CAD build for the part. Positions are in the model's coordinates, mm. A direction names the side the tool comes from. Coordinates: 2 decimals unless noted, no trailing zeros. Write each loop counter-clockwise with the first axis right and the second up, starting at its lowest first coordinate (ties: lowest second). Pieces come first, ordered by that corner, then holes. Notation, with made-up numbers: M 32.5,57.5 L 43.5,57.5 A19 cw 43.5,90.5 Z; hole C 52,47.25 d2. An arc over 180 degrees is marked long. Put each result on its own line as item: value. Start each with the question number.
Autodesk Inventor part; units mm, degrees
ref_plane "YZ Plane" through (0, 0, 0) normal (1, 0, 0) x (0, 1, 0)
ref_plane "XZ Plane" through (0, 0, 0) normal (0, 1, 0) x (-1, 0, 0)
ref_plane "XY Plane" through (0, 0, 0) normal (0, 0, 1) x (1, 0, 0)
sketch "Эскиз1" plane through (0, 0, 0) normal (1, 0, 0) x (0, 1, 0)
  line L0 (0, 0) -> (0, -73.7994) construction
  line L1 (23.5, 0) -> (23.5, -65.8206)
  line L2 (23.5, -65.8206) -> (67.6779, -115.777)
  line L3 (125, -110.9688) -> (125, -104.777)
  line L4 (125, -104.777) -> (67.2948, -104.777)
  line L5 (67.2948, -104.777) -> (40.0448, -73.9627)
  line L6 (27.5, -40.8401) -> (27.5, -5)
  line L7 (27.5, -5) -> (32.5, -5)
  line L8 (32.5, -5) -> (32.5, 0)
  line L9 (32.5, 0) -> (23.5, 0)
  line L10 (67.6779, -115.777) -> (90, -115.777)
  line L11 (90, -115.777) -> (90, -119.777)
  line L12 (90, -119.777) -> (125, -119.777)
  line L13 (125, -119.777) -> (125, -110.9688)
  arc A0 (27.5, -40.8401) -> (40.0448, -73.9627) centre (77.5, -40.8401) ccw
  point P0 (27.5, -59.777)
  point P1 (125, -98)
  dimension "d13" = 47
  dimension "d14" = 180
  dimension "d15" = 250
  dimension "d16" = 7
  dimension "d18" = 0
  dimension "d19" = 15
  dimension "d20" = 4
  dimension "d21" = 65
  dimension "d22" = 4
  dimension "d23" = 5
  dimension "d24" = 59.777
  dimension "d25" = 60
  dimension "d53" = 50
revolve "Вращение1" add sketch "Эскиз1" angle 360 about axis through (0, 0, 0) along (0, 0, -1)
sketch "Эскиз2" plane through (0, 0, -119.777) normal (0, 0, -1) x (-1, 0, 0)
  circle A0 centre (-41.139, 99.317) radius 8
  circle A1 centre (0, 0) radius 107.5
  circle A2 centre (-99.3174, 41.1381) radius 8
  circle A3 centre (-99.317, -41.139) radius 8
  circle A4 centre (-41.1381, -99.3174) radius 8
  circle A5 centre (41.139, -99.317) radius 8
  circle A6 centre (99.3174, -41.1381) radius 8
  circle A7 centre (99.317, 41.139) radius 8
  circle A8 centre (41.1381, 99.3174) radius 8
  dimension "d27" = 215
  dimension "d28" = 16
  dimension "d29" = 41.139
  dimension "d30" = 99.317
  dimension "d33" = 360
extrude "Выдавливание1" cut sketch "Эскиз2" against normal through all contours A0 A1 | A1 A0 | A8 A1 | A1 A8 | A2 A1 | A1 A2 | A7 A1 | A1 A7 | A3 A1 | A1 A3 | A4 A1 | A1 A4 | A6 A1 | A1 A6 | A5 A1 | A1 A5
thread "Резьба9"
thread "Резьба10"
thread "Резьба11"
thread "Резьба12"
thread "Резьба13"
thread "Резьба14"
thread "Резьба15"
thread "Резьба16"
properties part number "Крышка_быстроходного"
(1) Slice it at A-A, the plane x = 0. Write the cut outline in (y, z), then the cut area to 3 significant figures.
(2) Which spindle directions (+Z, -Z, +X, -X, +Y, -Y) get a long thin tool onto all of the face, cutting with end or side? Do faces 1 (the face through (-22, 9, 0)), 2 (the face through (-9.76, 31, -2.46)), 3 (the face through (7, -27, -5)), 4 (the face through (67, 13, -115.777)), 5 (the face through (-98.28, 49.07, -112.38)). Say none if no direction does.
(3) Slice it at D-D, the plane z = -26.5. Write the cut outline in (x, y), then the cut area to 3 significant figures.
(4) Drill centre lines: line 1 (X direction, y = 104, z = -111); line 2 (X direction, y = 31.5, z = -109); line 3 (Y direction, x = -18.5, z = -101). Where is each one in solid material? Low to high. Write a range as [from, to].
(5) Two-plate mould, pull along X, no slides. Class faces 6 (the face through (-54, 54, -104.777)), 7 (the face through (-39.405, -107.127, -112.382)), 8 (the face through (26.846, -5.961, -22.669)): +X half, -X half, draft (parallel to the pull), parting line (faces both ways), or undercut.
(6) Slice it at C-C, the plane x = -102. Write the cut outline in (y, z).
(7) Drop flat-ended pins along their axis: pin 1 (14.5 mm diameter, centred on x = 41.14, y = -99.32, fed in from -Z); pin 2 (5 mm diameter, centred on x = 10, z = -90.5, fed in from -Y); pin 3 (8 mm diameter, centred on y = -22.5, z = -101, fed in from -X); pin 4 (8 mm diameter, centred on x = 22, z = -15, fed in from -Y). Give the stop position or say it passes through.
Result set:
1. outline: M -125,-119.78 L -90,-119.78 L -90,-115.78 L -67.68,-115.78 L -23.5,-65.82 L -23.5,0 L -32.5,0 L -32.5,-5 L -27.5,-5 L -27.5,-40.84 A50 cw -40.04,-73.96 L -67.29,-104.78 L -125,-104.78 Z; M 23.5,-65.82 L 67.68,-115.78 L 90,-115.78 L 90,-119.78 L 125,-119.78 L 125,-104.78 L 67.29,-104.78 L 40.04,-73.96 A50 cw 27.5,-40.84 L 27.5,-5 L 32.5,-5 L 32.5,0 L 23.5,0 Z
1. area: 3,070 mm^2
2. face 1: +Z, +X, -X, +Y, -Y
2. face 2: +Z
2. face 3: none
2. face 4: -Z
2. face 5: +Z, -Z
3. outline: C 0,0 d55; hole C 0,0 d47
3. area: 641 mm^2
4. line 1: x = [-69.35, -47.62], [-34.65, 34.65], [47.63, 69.35]
4. line 2: x = [-120.97, -53.04], [53.04, 120.97]
4. line 3: y = [-61.22, -51.38], [51.38, 61.22]
5. face 6: draft
5. face 7: undercut
5. face 8: parting line
6. outline: M -72.26,-119.78 L -48.67,-119.78 L -48.67,-104.78 L -72.26,-104.78 Z; M -33.6,-119.78 L 33.6,-119.78 L 33.6,-104.78 L -33.6,-104.78 Z; M 48.68,-119.78 L 72.26,-119.78 L 72.26,-104.78 L 48.68,-104.78 Z
7. pin 1: passes through
7. pin 2: stops at y = -56.04
7. pin 3: stops at x = -123.19
7. pin 4: stops at y = -20.79
